Verification items for the finished model (mm, model axes). A direction names the side the tool comes from. Round coordinates to 2 decimals unless told otherwise and drop trailing zeros. Write each loop counter-clockwise with the first axis right and the second up, starting at its lowest first coordinate (ties: lowest second). Pieces come first, ordered by that corner, then holes. Notation, with made-up numbers: M -1.75,-11 L 56.25,-11 A11 ccw 56.25,5 Z; hole C 10.5,56.25 d9. An arc over 180 degrees is marked long. Answer in a Markdown table with one row per item. Add a question column.
1. Sectioned sample at A-A on y = 2. Record the cut outline in (x, z), plus the area to 3 significant figures.
2. Material ranges on probe 1 along Z at (x, y) = (4, 6.5); probe 2 along Y at (x, z) = (4.5, -3.4); probe 3 along X at (y, z) = (4.5, 3.5), recorded low to high.
3. Set-up check for faces 1 (the cylindrical face through (7.168, 0.493, 1.737)), 2 (the flat face through (7, 3.5, -3.5)): record each of +Z, -Z, +X, -X, +Y, -Y from which the full face is reachable in a straight line by a thin tool's end or side.
4. Draft check along Z on faces 3 (the flat face through (-4, 4, 10)), 4 (the cylindrical face through (-0.434, 0.493, -1.952)), 5 (the cylindrical face through (8.5, 0.5, 0)). Enter one of: pulls with the +Z half, pulls with the -Z half, needs draft (parallel to the pull), parting line crosses it, or undercut.
5. Sectioned sample at D-D on y = 4.5. Record the cut outline in (x, z).
6. Sectioned sample at B-B on x = 0. Record the cut outline in (y, z).
7. Sectioned sample at C-C on z = 0. Record the cut outline in (x, y), plus the area to 3 significant figures.
8. Go/stop test with flat-tipped pins: pin 1 Ø0.7 at (y, z) = (5, 8.5) entering from -X; pin 2 Ø0.5 at (y, z) = (4, -3) entering from -X; pin 3 Ø1.4 at (x, z) = (7, 0) entering from +Y; pin 4 Ø1 at (x, z) = (-7, 0) entering from -Y. Record where each tip stops, or that it passes through.
```python
from build123d import *

# Parameters (mm, degrees)
EXTRUDE1_DEPTH      = 4
EXTRUDE2_DEPTH      = 12.357816692
EXTRUDE2_DEPTH_BACK = 12.357816692
SKETCH2_R           = 1
EXTRUDE3_DEPTH      = 12.357816692
EXTRUDE3_DEPTH_BACK = 12.357816692
SKETCH4_W           = 6
SKETCH4_H           = 8.732029078
FILLET1_R           = 0.2
FILLET2_R           = 1
EXTRUDE4_DEPTH      = 14
EXTRUDE4_DEPTH_BACK = 3
SKETCH3_R           = 1.5
EXTRUDE5_DEPTH      = 9
SKETCH6_R           = 1.5
EXTRUDE6_DEPTH      = 1
SKETCH7_R           = 0.6
EXTRUDE7_DEPTH      = 1
FILLET3_R           = 1
SKETCH8_R           = 2
EXTRUDE8_DEPTH      = 1


with BuildPart() as part:
    # Sketch1 → Extrude1 (new, symmetric)
    with BuildSketch(Plane.XY):
        Polygon((0, 0), (-7, 0), (-7, 8), (7, 8), (7, 0), align=None)
    extrude(amount=EXTRUDE1_DEPTH, both=True)

    # Sketch2 → Extrude2 (cut, two sides: drawn at the far end of the back side and taken through both)
    with BuildSketch(Plane.XY.offset(-EXTRUDE2_DEPTH_BACK)):
        with Locations((4.5, 4.5)):
            Circle(SKETCH2_R)
    extrude(amount=EXTRUDE2_DEPTH + EXTRUDE2_DEPTH_BACK, mode=Mode.SUBTRACT)

    # Sketch4 → Extrude3 (cut, two sides: drawn at the far end of the back side and taken through both)
    with BuildSketch(Plane(origin=(0, 0, 0), x_dir=(0, 0, -1), z_dir=(1, 0, 0)).offset(-EXTRUDE3_DEPTH_BACK)):
        with Locations((0, 5.366014539)):
            Rectangle(SKETCH4_W, SKETCH4_H)
    extrude(amount=EXTRUDE3_DEPTH + EXTRUDE3_DEPTH_BACK, mode=Mode.SUBTRACT)

    # Fillet1
    fillet1_edges = [part.edges().sort_by_distance(p)[0] for p in [
        (0, 0, 4),
        (0, 0, -4),
    ]]
    fillet(fillet1_edges, radius=FILLET1_R)

    # Fillet2
    fillet2_edges = [part.edges().sort_by_distance(p)[0] for p in [
        (-7, 8, -3.5),
        (7, 8, -3.5),
        (-7, 8, 3.5),
        (7, 8, 3.5),
    ]]
    fillet(fillet2_edges, radius=FILLET2_R)

    # Sketch3 → Extrude4 (add, two sides: drawn at the far end of the back side and taken through both)
    with BuildSketch(Plane.XY.offset(-EXTRUDE4_DEPTH_BACK)):
        with Locations((-3, 4.5)):
            Circle(SKETCH3_R)
    extrude(amount=EXTRUDE4_DEPTH + EXTRUDE4_DEPTH_BACK)

    # Sketch5 → Extrude5 (cut)
    with BuildSketch(Plane.XY.offset(14)):
        Polygon((-4, 4.5), (-4, 6.060686456), (-4.95644391, 6.060686456), (-4.95644391, 2.5), (-4, 2.5), align=None)
    extrude(amount=-EXTRUDE5_DEPTH, mode=Mode.SUBTRACT)

    # Sketch6 → Extrude6 (add)
    with BuildSketch(Plane.XZ):
        with Locations((-7, 0)):
            Circle(SKETCH6_R)
        with Locations((7, 0)):
            Circle(SKETCH6_R)
    extrude(amount=-EXTRUDE6_DEPTH)

    # Sketch7 → Extrude7 (cut)
    with BuildSketch(Plane.XZ):
        with Locations((-7, 0)):
            Circle(SKETCH7_R)
        with Locations((7, 0)):
            Circle(SKETCH7_R)
    extrude(amount=-EXTRUDE7_DEPTH, mode=Mode.SUBTRACT)

    # Fillet3
    fillet3_edges = [part.edges().sort_by_distance(p)[0] for p in [
        (7, 0.5, -1.5),
        (7, 0.5, 1.5),
        (-7, 0.5, 1.5),
        (-7, 0.5, -1.5),
    ]]
    fillet(fillet3_edges, radius=FILLET3_R)

    # Sketch8 → Extrude8 (cut)
    with BuildSketch(Plane.XZ):
        Circle(SKETCH8_R)
    extrude(amount=-EXTRUDE8_DEPTH, mode=Mode.SUBTRACT)


solid = part.part
```
Geometry check:
| question | item | result |
|---|---|---|
| 1 | outline | M -7,-4 L 7,-4 L 7,-3 L -7,-3 Z; M -7,3 L 7,3 L 7,4 L -7,4 Z |
| 1 | area | 28.0 mm2 |
| 2 | probe 1 | z = -4 to -3, 3 to 4 |
| 2 | probe 2 | y = 0 to 3.5, 5.5 to 8 |
| 2 | probe 3 | x = -7 to 3.5, 5.5 to 7 |
| 3 | face 1 | +Z, +X, +Y, -Y |
| 3 | face 2 | -Z, +X, +Y, -Y |
| 4 | face 3 | needs draft |
| 4 | face 4 | undercut |
| 4 | face 5 | parting line crosses it |
| 5 | outline | M -7,-4 L 3.5,-4 L 3.5,-3 L -1.5,-3 L -1.5,3 L 3.5,3 L 3.5,4 L -1.5,4 L -1.5,14 L -4,14 L -4,5 L -4.5,5 L -4.5,4 L -7,4 L -7,3 L -4.5,3 L -4.5,-3 L -7,-3 Z; M 5.5,-4 L 7,-4 L 7,-3 L 5.5,-3 Z; M 5.5,3 L 7,3 L 7,4 L 5.5,4 Z |
| 6 | outline | M 0,-3.8 A0.2 ccw 0.2,-4 L 8,-4 L 8,-3 L 1,-3 L 1,-2 L 0,-2 Z; M 0,2 L 1,2 L 1,3 L 8,3 L 8,4 L 0.2,4 A0.2 ccw 0,3.8 Z |
| 7 | outline | M -8.5,0 L -7.6,0 L -7.6,1 L -8.5,1 Z; M -6.4,0 L -2,0 L -2,1 L -6.4,1 Z; C -3,4.5 d3; M 2,0 L 6.4,0 L 6.4,1 L 2,1 Z; M 7.6,0 L 8.5,0 L 8.5,1 L 7.6,1 Z |
| 7 | area | 17.7 mm2 |
| 8 | pin 1 | stops at x = -4 |
| 8 | pin 2 | stops at x = -7 |
| 8 | pin 3 | stops at y = 1 |
| 8 | pin 4 | passes through |
